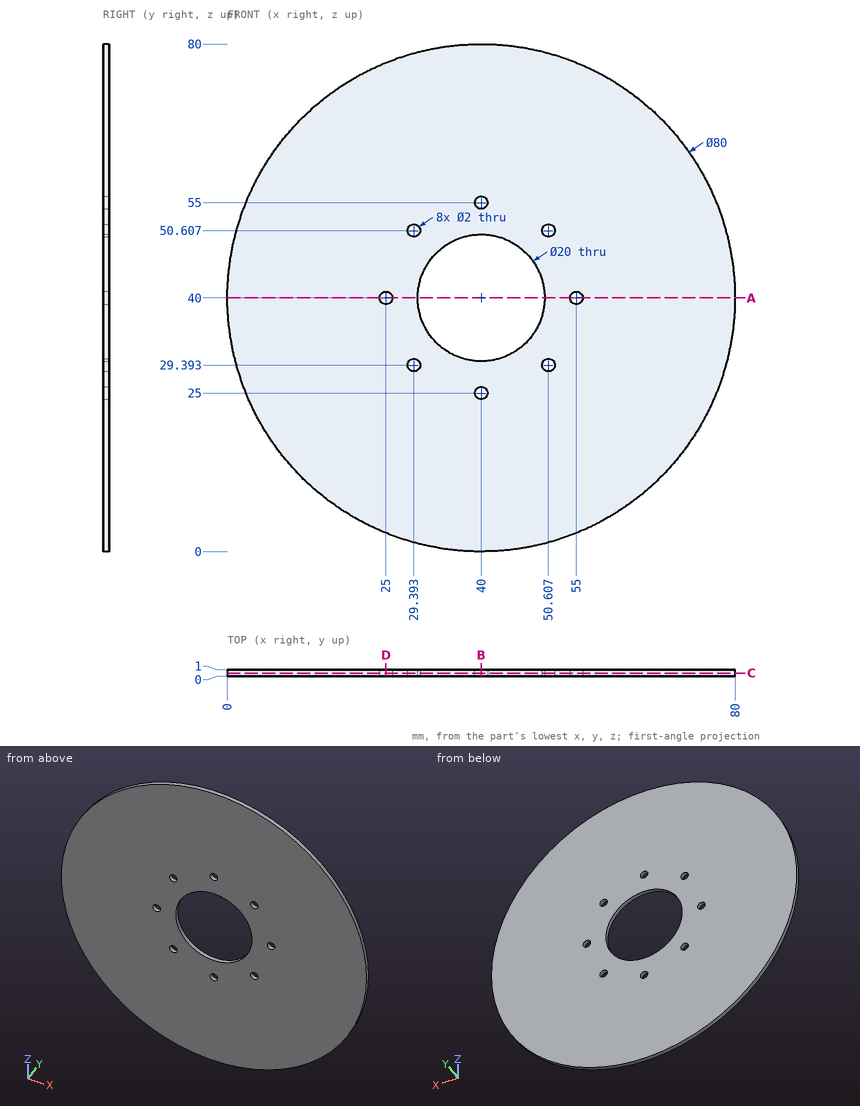
The figure shows three views and two pictorial views of one solid part (mm, origin at its lowest corner). Answer the questions. Give positions to 0.01 mm unless a question says otherwise; leave off trailing zeros. Loops run counter-clockwise (first coordinate to the right, second up) from the corner with the lowest first, then second, coordinate; pieces in that order, holes last. Notation, with made-up numbers: M 58,-11.5 L 82,-11.5 A22 cw 82,1.5 Z; hole C -10.75,71.5 d7. An arc over 180 degrees is marked long. Write each question's results on one line, items separated by ' | '.
1. Section A-A on z = 40 is taken. Give the vertices of the cut face in (x, y).
Values:
outline: M 0,0 L 24,0 L 24,1 L 0,1 Z; M 26,0 L 30,0 L 30,1 L 26,1 Z; M 50,0 L 54,0 L 54,1 L 50,1 Z; M 56,0 L 80,0 L 80,1 L 56,1 Z
2. Section C-C on y = 0.45 is taken. State how many separate pieces and enclosed holes the cut face has, plus the area to 3 significant figures.
Values:
separate pieces: 1 | enclosed holes: 9 | area: 4,690 mm^2
3. Section D-D on x = 25 is taken. Give the vertices of the cut face in (y, z).
Values:
outline: M 0,2.92 L 1,2.92 L 1,39 L 0,39 Z; M 0,41 L 1,41 L 1,77.08 L 0,77.08 Z
4. Given pin 1 (1.2 mm diameter, centred on x = 50.61, z = 50.61, fed in from -Y), flat-ended and moving along its own axis, determine where the tip first touches the part or whether it passes through.
Values:
pin 1: passes through
5. Section B-B on x = 40 is taken. Give the vertices of the cut face in (y, z).
Values:
outline: M 0,0 L 1,0 L 1,24 L 0,24 Z; M 0,26 L 1,26 L 1,30 L 0,30 Z; M 0,50 L 1,50 L 1,54 L 0,54 Z; M 0,56 L 1,56 L 1,80 L 0,80 Z
6. Straight lines are drawn through the part: line 1 (X direction, y = 0.75, z = 40); line 2 (Z direction, x = 50.5, y = 0.35); line 3 (X direction, y = 0.1, z = 31) (1 decimal). For each, find the intervals that lie inside material, in ascending order. Write a range as [from, to].
Values:
line 1: x = [0, 24], [26, 30], [50, 54], [56, 80] | line 2: z = [1.4, 28.4], [30.39, 49.61], [51.6, 78.6] | line 3: x = [1, 35.6], [44.4, 79]
